Autodesk Inventor part; units mm, degrees
ref_plane "YZ Plane" through (0, 0, 0) normal (1, 0, 0) x (0, 1, 0)
ref_plane "XZ Plane" through (0, 0, 0) normal (0, 1, 0) x (-1, 0, 0)
ref_plane "XY Plane" through (0, 0, 0) normal (0, 0, 1) x (1, 0, 0)
sketch "Sketch1" plane through (0, 0, 0) normal (0, 0, 1) x (1, 0, 0)
  line L0 (57.15, -19.05) -> (-57.15, -19.05)
  line L1 (-57.15, -19.05) -> (-57.15, 19.05)
  line L2 (-57.15, 19.05) -> (57.15, 19.05)
  line L3 (57.15, 19.05) -> (57.15, -19.05)
  line L4 (57.15, -19.05) -> (-57.15, 19.05) construction
  line L5 (-57.15, -19.05) -> (57.15, 19.05) construction
  point P0 (0, 0)
  dimension "d0" = 114.3
  dimension "d1" = 38.1
extrude "Extrusion1" add sketch "Sketch1" along normal blind 6.35
sketch "Sketch2" plane through (0, 0, 6.35) normal (0, 0, 1) x (1, 0, 0)
  line L0 (-57.15, 19.05) -> (-57.15, -19.05)
  line L1 (57.15, 19.05) -> (-57.15, 19.05)
  point P0 (0, 0)
  point P1 (-44.45, 6.35)
  point P2 (-31.75, 6.35)
  point P3 (-19.05, 6.35)
  point P4 (-57.15, 0)
  dimension "d5" = 12.7
  dimension "d6" = 12.7
  dimension "d14" = 12.7
  dimension "d15" = 12.7
hole "Hole1" at (-44.45, 6.35, 6.35) at (-31.75, 6.35, 6.35) at (-19.05, 6.35, 6.35) direction (0, 0, -1) diameter 3.9624 end through all
sketch "Sketch3" plane through (0, 0, 6.35) normal (0, 0, 1) x (1, 0, 0)
  line L0 (57.15, 19.05) -> (-57.15, 19.05)
  line L1 (-57.15, -19.05) -> (57.15, -19.05)
  line L2 (57.15, -19.05) -> (57.15, 19.05)
  point P0 (0, 0)
  point P1 (53.975, 12.7)
  point P2 (53.975, -12.7)
  dimension "d16" = 6.35
  dimension "d17" = 6.35
  dimension "d18" = 3.175
hole "Hole2" at (53.975, 12.7, 6.35) at (53.975, -12.7, 6.35) direction (0, 0, -1) diameter 4.318 end through all
sketch "Sketch5" plane through (0, 0, 6.35) normal (0, 0, 1) x (1, 0, 0)
  line L0 (57.15, -19.05) -> (57.15, 19.05) construction
  line L1 (6.35, 0) -> (31.75, 0) construction
  point P0 (0, 0)
  point P1 (57.15, 0)
  point P2 (19.05, 0)
  dimension "d28" = 25.4
  dimension "d37" = 38.1
hole "Hole3" at (6.35, 0, 6.35) at (31.75, 0, 6.35) direction (0, 0, -1) diameter 3.9624 end through all
properties part number "EL2-014" material "Aluminum 6061"
Verification items for the finished model (mm, model axes). Coordinates: 2 decimals unless noted, no trailing zeros. Order: outer loops, then holes, each group sorted by start corner. A loop starts at its lowest first (then second) coordinate and runs counter-clockwise, first axis right, second up. Notation, with made-up numbers: (89.25, 69) -> (109.25, 69) arc R6 cw to (109.25, 76) -> close; hole circle Ø5 at (30.5, -40). An arc over 180 degrees is marked (long way). Put each result on its own line as item: value. Start each with the question number.
1. Mould release check, pull along X, two halves, no side actions. Record for faces 1 (the flat face through (-57.15, 0, 3)), 2 (the cylindrical face through (30.1, -1.1, 3.1)), 3 (the flat face through (-1, 0, 6.35)): released by +X, released by -X, zero draft, split by the parting line, or undercut.
2. Material ranges on L1, parallel to X at y = 0, z = 4.75; L2, parallel to X at y = 6.35, z = 3.75; L3, parallel to Y at x = 31.75, z = 4.5, recorded low to high. Write a range as [from, to].
3. Cross-section at A-A, the plane y = 12.7. Record the boundary of the cut face in (x, z), then the cut area to 3 significant figures.
4. Cross-section at B-B, the plane x = -31.75. Record the boundary of the cut face in (y, z), then the cut area to 3 significant figures.
5. Cross-section at C-C, the plane z = 4.75. Record the boundary of the cut face in (x, y) (3 decimals).
6. Cross-section at D-D, the plane y = 0. Record the boundary of the cut face in (x, z), then the cut area to 3 significant figures.
Computed:
1. face 1: released by -X
1. face 2: undercut
1. face 3: zero draft
2. L1: [-57.15, 4.37], [8.33, 29.77], [33.73, 57.15]
2. L2: [-57.15, -46.43], [-42.47, -33.73], [-29.77, -21.03], [-17.07, 57.15]
2. L3: [-19.05, -1.98], [1.98, 19.05]
3. outline: (-57.15, 0) -> (51.82, 0) -> (51.82, 6.35) -> (-57.15, 6.35) -> close; (56.13, 0) -> (57.15, 0) -> (57.15, 6.35) -> (56.13, 6.35) -> close
3. area: 698 mm2
4. outline: (-19.05, 0) -> (4.37, 0) -> (4.37, 6.35) -> (-19.05, 6.35) -> close; (8.33, 0) -> (19.05, 0) -> (19.05, 6.35) -> (8.33, 6.35) -> close
4. area: 217 mm2
5. outline: (-57.15, -19.05) -> (57.15, -19.05) -> (57.15, 19.05) -> (-57.15, 19.05) -> close; hole circle Ø3.962 at (-44.45, 6.35); hole circle Ø3.962 at (-31.75, 6.35); hole circle Ø3.962 at (-19.05, 6.35); hole circle Ø3.962 at (6.35, 0); hole circle Ø3.962 at (31.75, 0); hole circle Ø4.318 at (53.975, -12.7); hole circle Ø4.318 at (53.975, 12.7)
6. outline: (-57.15, 0) -> (4.37, 0) -> (4.37, 6.35) -> (-57.15, 6.35) -> close; (8.33, 0) -> (29.77, 0) -> (29.77, 6.35) -> (8.33, 6.35) -> close; (33.73, 0) -> (57.15, 0) -> (57.15, 6.35) -> (33.73, 6.35) -> close
6. area: 675 mm2
